CAD build for the part. Positions are in the model's coordinates, mm. Give positions to 0.01 mm unless a question says otherwise; leave off trailing zeros. Answer as a JSON object with one key per item and string values.
from build123d import *

# Parameters (mm, degrees)
MODEL_R         = 2.5
EXTRUDE_1_DEPTH = 305


with BuildPart() as part:
    # Model → Бобышка-Вытянуть1 (new body)
    with BuildSketch(Plane.XY):
        with BuildLine():
            Line((18.94214915, 33.362214718), (18.94214915, 34.923300122))
            ThreePointArc((18.94214915, 34.923300122), (18.789908215, 35.688666987), (18.356362712, 36.337513684))
            Line((18.356362712, 36.337513684), (16.662250163, 38.031626234))
            ThreePointArc((16.662250163, 38.031626234), (16.337826814, 38.248398985), (15.955143382, 38.324519453))
            Line((15.955143382, 38.324519453), (15.14214915, 38.324519453))
            ThreePointArc((15.14214915, 38.324519453), (15.000727794, 38.265940809), (14.94214915, 38.124519453))
            Line((14.94214915, 38.124519453), (14.94214915, 36.354519453))
            ThreePointArc((14.94214915, 36.354519453), (14.787820008, 36.12354957), (14.515372455, 36.177742757))
            Line((14.515372455, 36.177742757), (13.015372455, 37.677742757))
            ThreePointArc((13.015372455, 37.677742757), (12.961179267, 37.758848595), (12.94214915, 37.854519453))
            Line((12.94214915, 37.854519453), (12.94214915, 41.524519453))
            ThreePointArc((12.94214915, 41.524519453), (13.381488978, 42.585179625), (14.44214915, 43.024519453))
            Line((14.44214915, 43.024519453), (18.11214915, 43.024519453))
            ThreePointArc((18.11214915, 43.024519453), (18.207820008, 43.005489336), (18.288925845, 42.951296148))
            Line((18.288925845, 42.951296148), (19.788925845, 41.451296148))
            ThreePointArc((19.788925845, 41.451296148), (19.843119033, 41.178848595), (19.61214915, 41.024519453))
            Line((19.61214915, 41.024519453), (17.84214915, 41.024519453))
            ThreePointArc((17.84214915, 41.024519453), (17.700727794, 40.965940809), (17.64214915, 40.824519453))
            Line((17.64214915, 40.824519453), (17.64214915, 40.011525221))
            ThreePointArc((17.64214915, 40.011525221), (17.718269617, 39.628841789), (17.935042369, 39.30441844))
            Line((17.935042369, 39.30441844), (19.629154919, 37.61030589))
            ThreePointArc((19.629154919, 37.61030589), (20.278001616, 37.176760388), (21.043368481, 37.024519453))
            Line((21.043368481, 37.024519453), (22.604453885, 37.024519453))
            ThreePointArc((22.604453885, 37.024519453), (22.687205621, 37.010426533), (22.760627647, 36.969736655))
            Line((22.760627647, 36.969736655), (22.94214915, 36.824519453))
            Line((22.94214915, 36.824519453), (23.123670653, 36.969736655))
            ThreePointArc((23.123670653, 36.969736655), (23.197092679, 37.010426533), (23.279844415, 37.024519453))
            Line((23.279844415, 37.024519453), (24.840929819, 37.024519453))
            ThreePointArc((24.840929819, 37.024519453), (25.606296684, 37.176760388), (26.255143382, 37.61030589))
            Line((26.255143382, 37.61030589), (27.949255931, 39.30441844))
            ThreePointArc((27.949255931, 39.30441844), (28.166028683, 39.628841789), (28.24214915, 40.011525221))
            Line((28.24214915, 40.011525221), (28.24214915, 40.824519453))
            ThreePointArc((28.24214915, 40.824519453), (28.183570506, 40.965940809), (28.04214915, 41.024519453))
            Line((28.04214915, 41.024519453), (26.27214915, 41.024519453))
            ThreePointArc((26.27214915, 41.024519453), (26.041179267, 41.178848595), (26.095372455, 41.451296148))
            Line((26.095372455, 41.451296148), (27.595372455, 42.951296148))
            ThreePointArc((27.595372455, 42.951296148), (27.676478292, 43.005489336), (27.77214915, 43.024519453))
            Line((27.77214915, 43.024519453), (31.44214915, 43.024519453))
            ThreePointArc((31.44214915, 43.024519453), (32.502809322, 42.585179625), (32.94214915, 41.524519453))
            Line((32.94214915, 41.524519453), (32.94214915, 37.854519453))
            ThreePointArc((32.94214915, 37.854519453), (32.923119033, 37.758848595), (32.868925845, 37.677742757))
            Line((32.868925845, 37.677742757), (31.368925845, 36.177742757))
            ThreePointArc((31.368925845, 36.177742757), (31.096478292, 36.12354957), (30.94214915, 36.354519453))
            Line((30.94214915, 36.354519453), (30.94214915, 38.124519453))
            ThreePointArc((30.94214915, 38.124519453), (30.883570506, 38.265940809), (30.74214915, 38.324519453))
            Line((30.74214915, 38.324519453), (29.929154919, 38.324519453))
            ThreePointArc((29.929154919, 38.324519453), (29.546471486, 38.248398985), (29.222048137, 38.031626234))
            Line((29.222048137, 38.031626234), (27.527935588, 36.337513684))
            ThreePointArc((27.527935588, 36.337513684), (27.094390085, 35.688666987), (26.94214915, 34.923300122))
            Line((26.94214915, 34.923300122), (26.94214915, 33.362214718))
            ThreePointArc((26.94214915, 33.362214718), (26.92805623, 33.279462982), (26.887366352, 33.206040956))
            Line((26.887366352, 33.206040956), (26.74214915, 33.024519453))
            Line((26.74214915, 33.024519453), (26.887366352, 32.84299795))
            ThreePointArc((26.887366352, 32.84299795), (26.92805623, 32.769575923), (26.94214915, 32.686824188))
            Line((26.94214915, 32.686824188), (26.94214915, 31.125738784))
            ThreePointArc((26.94214915, 31.125738784), (27.094390085, 30.360371919), (27.527935588, 29.711525221))
            Line((27.527935588, 29.711525221), (29.222048137, 28.017412672))
            ThreePointArc((29.222048137, 28.017412672), (29.546471486, 27.80063992), (29.929154919, 27.724519453))
            Line((29.929154919, 27.724519453), (30.74214915, 27.724519453))
            ThreePointArc((30.74214915, 27.724519453), (30.883570506, 27.783098097), (30.94214915, 27.924519453))
            Line((30.94214915, 27.924519453), (30.94214915, 29.694519453))
            ThreePointArc((30.94214915, 29.694519453), (31.096478292, 29.925489336), (31.368925845, 29.871296148))
            Line((31.368925845, 29.871296148), (32.868925845, 28.371296148))
            ThreePointArc((32.868925845, 28.371296148), (32.923119033, 28.290190311), (32.94214915, 28.194519453))
            Line((32.94214915, 28.194519453), (32.94214915, 24.524519453))
            ThreePointArc((32.94214915, 24.524519453), (32.502809322, 23.463859281), (31.44214915, 23.024519453))
            Line((31.44214915, 23.024519453), (27.77214915, 23.024519453))
            ThreePointArc((27.77214915, 23.024519453), (27.676478292, 23.04354957), (27.595372455, 23.097742757))
            Line((27.595372455, 23.097742757), (26.095372455, 24.597742757))
            ThreePointArc((26.095372455, 24.597742757), (26.041179267, 24.870190311), (26.27214915, 25.024519453))
            Line((26.27214915, 25.024519453), (28.04214915, 25.024519453))
            ThreePointArc((28.04214915, 25.024519453), (28.183570506, 25.083098097), (28.24214915, 25.224519453))
            Line((28.24214915, 25.224519453), (28.24214915, 26.037513684))
            ThreePointArc((28.24214915, 26.037513684), (28.166028683, 26.420197117), (27.949255931, 26.744620465))
            Line((27.949255931, 26.744620465), (26.255143382, 28.438733015))
            ThreePointArc((26.255143382, 28.438733015), (25.606296684, 28.872278518), (24.840929819, 29.024519453))
            Line((24.840929819, 29.024519453), (23.279844415, 29.024519453))
            ThreePointArc((23.279844415, 29.024519453), (23.197092679, 29.038612373), (23.123670653, 29.07930225))
            Line((23.123670653, 29.07930225), (22.94214915, 29.224519453))
            Line((22.94214915, 29.224519453), (22.760627647, 29.07930225))
            ThreePointArc((22.760627647, 29.07930225), (22.687205621, 29.038612373), (22.604453885, 29.024519453))
            Line((22.604453885, 29.024519453), (21.043368481, 29.024519453))
            ThreePointArc((21.043368481, 29.024519453), (20.278001616, 28.872278518), (19.629154919, 28.438733015))
            Line((19.629154919, 28.438733015), (17.935042369, 26.744620465))
            ThreePointArc((17.935042369, 26.744620465), (17.718269617, 26.420197117), (17.64214915, 26.037513684))
            Line((17.64214915, 26.037513684), (17.64214915, 25.224519453))
            ThreePointArc((17.64214915, 25.224519453), (17.700727794, 25.083098097), (17.84214915, 25.024519453))
            Line((17.84214915, 25.024519453), (19.61214915, 25.024519453))
            ThreePointArc((19.61214915, 25.024519453), (19.843119033, 24.870190311), (19.788925845, 24.597742757))
            Line((19.788925845, 24.597742757), (18.288925845, 23.097742757))
            ThreePointArc((18.288925845, 23.097742757), (18.207820008, 23.04354957), (18.11214915, 23.024519453))
            Line((18.11214915, 23.024519453), (14.44214915, 23.024519453))
            ThreePointArc((14.44214915, 23.024519453), (13.381488978, 23.463859281), (12.94214915, 24.524519453))
            Line((12.94214915, 24.524519453), (12.94214915, 28.194519453))
            ThreePointArc((12.94214915, 28.194519453), (12.961179267, 28.290190311), (13.015372455, 28.371296148))
            Line((13.015372455, 28.371296148), (14.515372455, 29.871296148))
            ThreePointArc((14.515372455, 29.871296148), (14.787820008, 29.925489336), (14.94214915, 29.694519453))
            Line((14.94214915, 29.694519453), (14.94214915, 27.924519453))
            ThreePointArc((14.94214915, 27.924519453), (15.000727794, 27.783098097), (15.14214915, 27.724519453))
            Line((15.14214915, 27.724519453), (15.955143382, 27.724519453))
            ThreePointArc((15.955143382, 27.724519453), (16.337826814, 27.80063992), (16.662250163, 28.017412672))
            Line((16.662250163, 28.017412672), (18.356362712, 29.711525221))
            ThreePointArc((18.356362712, 29.711525221), (18.789908215, 30.360371919), (18.94214915, 31.125738784))
            Line((18.94214915, 31.125738784), (18.94214915, 32.686824188))
            ThreePointArc((18.94214915, 32.686824188), (18.95624207, 32.769575923), (18.996931948, 32.84299795))
            Line((18.996931948, 32.84299795), (19.14214915, 33.024519453))
            Line((19.14214915, 33.024519453), (18.996931948, 33.206040956))
            ThreePointArc((18.996931948, 33.206040956), (18.95624207, 33.279462982), (18.94214915, 33.362214718))
        make_face()
        with Locations((22.94214915, 33.024519453)):
            Circle(MODEL_R, mode=Mode.SUBTRACT)
    extrude(amount=EXTRUDE_1_DEPTH)


solid = part.part
Item 1: Probe line 1 (X direction, y = 40.5, z = 41); line 2 (X direction, y = 39.5, z = 88); line 3 (X direction, y = 36.25, z = 170). List the from-to ranges inside material, lowest first. Write a range as from..to.
Entries:
{"line 1": "12.94..17.64, 28.24..32.94", "line 2": "12.94..17.78, 28.1..32.94", "line 3": "14.44..14.92, 18.44..27.45, 30.97..31.44"}
Item 2: Mould opens along Y. For faces 1 (the cylindrical face through (25.327, 33.775, 150.365)), 2 (the flat face through (25, 31, 0)) say: +Y half, -Y half, draft (parallel to the pull), parting line (faces both ways), or undercut.
Entries:
{"face 1": "undercut", "face 2": "draft"}
Item 3: Flat gauge pins, fed straight in: P1, Ø4, axis at x = 20.5, z = 258.5, coming from the +Y side; P2, Ø0.9, axis at y = 29, z = 132.5, coming from the -X side; P3, Ø1.7, axis at x = 24.5, z = 172, coming from the -Y side. Where does each tip first touch, or does it go through?
Entries:
{"P1": "y = 42.74", "P2": "x = 13.19", "P3": "y = 28.96"}
